The listing builds one solid part. Answer for the finished solid, in the listing's coordinates (mm). Coordinates: 2 decimals unless noted, no trailing zeros. Write each loop counter-clockwise with the first axis right and the second up, starting at its lowest first coordinate (ties: lowest second). Pieces come first, ordered by that corner, then holes. Notation, with made-up numbers: M -21.5,20 L 13.5,20 A30 cw 13.5,46 Z; hole C -5.75,17.5 d8. An arc over 180 degrees is marked long. Answer as CSV lines item,"result".
```python
from build123d import *

# Parameters (mm, degrees)
SKETCH1_R           = 2.0701
BOSS_EXTRUDE1_DEPTH = 2.286


with BuildPart() as part:
    # Sketch1 → Boss-Extrude1 (new body)
    with BuildSketch(Plane.XY.offset(2.286)):
        with BuildLine():
            Line((32.867737403, 47.774962564), (29.814450322, 47.774962564))
            Line((29.814450322, 47.774962564), (-12.7, 5.260512242))
            Line((-12.7, 5.260512242), (-12.7, -54.864))
            Line((-12.7, -54.864), (-10.541, -57.023))
            Line((-10.541, -57.023), (10.541, -57.023))
            Line((10.541, -57.023), (12.7, -54.864))
            Line((12.7, -54.864), (12.7, -7.890768363))
            ThreePointArc((12.7, -7.890768363), (13.183364969, -5.460728568), (14.559871939, -3.400640303))
            Line((14.559871939, -3.400640303), (47.774962564, 29.814450322))
            Line((47.774962564, 29.814450322), (47.774962564, 32.867737403))
            Line((47.774962564, 32.867737403), (32.867737403, 47.774962564))
        make_face()
        with Locations((35.921024484, 35.921024484)):
            Circle(SKETCH1_R, mode=Mode.SUBTRACT)
        with Locations((17.960512242, 17.960512242)):
            Circle(SKETCH1_R, mode=Mode.SUBTRACT)
        with Locations((8.980256121, 8.980256121)):
            Circle(SKETCH1_R, mode=Mode.SUBTRACT)
        with Locations((26.940768363, 26.940768363)):
            Circle(SKETCH1_R, mode=Mode.SUBTRACT)
        with Locations((0, -50.8)):
            Circle(SKETCH1_R, mode=Mode.SUBTRACT)
        with Locations((0, -25.4)):
            Circle(SKETCH1_R, mode=Mode.SUBTRACT)
        with Locations((0, -12.7)):
            Circle(SKETCH1_R, mode=Mode.SUBTRACT)
        with Locations((0, -38.1)):
            Circle(SKETCH1_R, mode=Mode.SUBTRACT)
        Circle(SKETCH1_R, mode=Mode.SUBTRACT)
    extrude(amount=-BOSS_EXTRUDE1_DEPTH)


solid = part.part
```
Q1. Find section A-A (y = -38.1). Give the vertices of the cut face in (x, z), and give its area (3 significant figures).
Output:
outline,"M -12.7,0 L -2.07,0 L -2.07,2.29 L -12.7,2.29 Z; M 2.07,0 L 12.7,0 L 12.7,2.29 L 2.07,2.29 Z"
area,"48.6 mm2"
Q2. Straight lines are drawn through the part: line 1 (Y direction, x = 0, z = 0.85); line 2 (Y direction, x = 32.5, z = 0.9); line 3 (X direction, y = -21.5, z = 0.8). For each, find the intervals that lie inside material, in ascending order.
Output:
line 1,"-57.02 to -52.87, -48.73 to -40.17, -36.03 to -27.47, -23.33 to -14.77, -10.63 to -2.07, 2.07 to 17.96"
line 2,"14.54 to 47.77"
line 3,"-12.7 to 12.7"
Q3. Find section B-B (x = 1). Give the vertices of the cut face in (y, z).
Output:
outline,"M -57.02,0 L -52.61,0 L -52.61,2.29 L -57.02,2.29 Z; M -48.99,0 L -39.91,0 L -39.91,2.29 L -48.99,2.29 Z; M -36.29,0 L -27.21,0 L -27.21,2.29 L -36.29,2.29 Z; M -23.59,0 L -14.51,0 L -14.51,2.29 L -23.59,2.29 Z; M -10.89,0 L -1.81,0 L -1.81,2.29 L -10.89,2.29 Z; M 1.81,0 L 18.96,0 L 18.96,2.29 L 1.81,2.29 Z"
Q4. The mould has two halves that part along X. Classify faces 1 (the flat face through (8.855, 26.815, 1.159)), 2 (the flat face through (40.426, 40.217, 1.159)), 3 (the cylindrical face through (-0.269, -23.348, 1.159)): pulls with the +X half, pulls with the -X half, needs draft (parallel to the pull), parting line crosses it, or undercut.
Output:
face 1,"pulls with the -X half"
face 2,"pulls with the +X half"
face 3,"undercut"
Q5. Find section C-C (z = 0.95). Count the separate pieces of the cut face and the enclosed holes in it, and give its area (3 significant figures).
Output:
separate pieces,"1"
enclosed holes,"9"
area,"2,770 mm2"
Q6. Flat-ended cylindrical pins translate along their axes: pin 1 Ø3.5 at (x, y) = (0, -50.8) entering from +Z; pin 2 Ø6.5 at (x, y) = (0, 0) entering from +Z. Find the tip coordinate at first contact, or state that the pin passes through.
Output:
pin 1,"through"
pin 2,"z = 2.29"
Q7. Find section D-D (y = 0). Give the vertices of the cut face in (x, z).
Output:
outline,"M -12.7,0 L -2.07,0 L -2.07,2.29 L -12.7,2.29 Z; M 2.07,0 L 17.96,0 L 17.96,2.29 L 2.07,2.29 Z"
